Could you check a few things on this model? Use its own coordinates, in mm. Give positions to 0.01 mm unless a question says otherwise; leave off trailing zeros. Loops run counter-clockwise (first coordinate to the right, second up) from the corner with the lowest first, then second, coordinate; pieces in that order, holes last. Notation, with made-up numbers: M 50.25,9.5 L 72.25,9.5 A18 cw 72.25,21.5 Z; hole C 59.5,89.5 d4. An arc over 180 degrees is marked long. Return JSON: item names as keys, results as strings. Group by question number.
1. For pin 1 (3 mm diameter, centred on x = 4, y = 2.5, fed in from +Z); pin 2 (1.9 mm diameter, centred on y = 2.5, z = -3.5, fed in from -X); pin 3 (2 mm diameter, centred on y = 3, z = -106, fed in from +X); pin 4 (6.5 mm diameter, centred on x = 12.7, z = -203.2, fed in from +Y), each with a flat end and sliding along its axis, tell me the tip position at first contact or that it passes through.
2. If we section it at B-B (z = -111): Write out the boundary of the cut face in (x, y).
3. If we section it at C-C (x = 82): Write out the boundary of the cut face in (y, z).
4. If we section it at A-A (x = 12.7): Write out the boundary of the cut face in (y, z).
5. Please list where these lines run through material, in increasing order: line 1 (Z direction, x = 12.7, y = 2.5); line 2 (X direction, y = 5.5, z = -37); line 3 (Z direction, x = 57, y = 5.25).
```python
from build123d import *

# Parameters (mm, degrees)
SKETCH1_W           = 95.25
SKETCH1_H           = 215.9
BOSS_EXTRUDE1_DEPTH = 6.35
SKETCH2_W           = 6.35
SKETCH2_H           = 12.7
CUT_EXTRUDE1_DEPTH  = 7.35
LPATTERN1_COUNT     = 10
LPATTERN1_PITCH     = 25.4
SKETCH3_W           = 12.7
SKETCH3_H           = 6.35
CUT_EXTRUDE2_DEPTH  = 7.35
LPATTERN2_COUNT     = 2
LPATTERN2_PITCH     = 25.4
LPATTERN2_COL_COUNT = 3
LPATTERN2_COL_PITCH = 25.4
SKETCH4_R           = 3.571875
CUT_EXTRUDE3_DEPTH  = 7.35


with BuildPart() as part:
    # Sketch1 → Boss-Extrude1 (new body)
    with BuildSketch(Plane(origin=(0, 0, 0), x_dir=(1, 0, 0), z_dir=(0, 1, 0))):
        with Locations((47.625, 107.95)):
            Rectangle(SKETCH1_W, SKETCH1_H)
    extrude(amount=BOSS_EXTRUDE1_DEPTH)

    # Sketch2 → Cut-Extrude1 (cut, through all)
    with BuildSketch(Plane(origin=(0, 6.35, 0), x_dir=(1, 0, 0), z_dir=(0, 1, 0))):
        with Locations((3.175, 209.55)):
            Rectangle(SKETCH2_W, SKETCH2_H)
        with Locations((92.075, 209.55)):
            Rectangle(SKETCH2_W, SKETCH2_H)
    cut_extrude1 = extrude(amount=-CUT_EXTRUDE1_DEPTH, mode=Mode.SUBTRACT)

    # LPattern1: Cut-Extrude1 ×10
    with Locations(*[(0, 0, i * LPATTERN1_PITCH) for i in range(1, LPATTERN1_COUNT)]):
        add(cut_extrude1, mode=Mode.SUBTRACT)

    # Sketch3 → Cut-Extrude2 (cut, through all)
    with BuildSketch(Plane(origin=(0, 6.35, 0), x_dir=(1, 0, 0), z_dir=(0, 1, 0))):
        with Locations((34.925, 212.725)):
            Rectangle(SKETCH3_W, SKETCH3_H)
    cut_extrude2 = extrude(amount=-CUT_EXTRUDE2_DEPTH, mode=Mode.SUBTRACT)

    # LPattern2: Cut-Extrude2 ×2
    with Locations(*[(-i * LPATTERN2_PITCH, 0, 0) for i in range(1, LPATTERN2_COUNT)]):
        add(cut_extrude2, mode=Mode.SUBTRACT)

    # LPattern2 col: Cut-Extrude2 ×3
    with Locations(*[(i * LPATTERN2_COL_PITCH, 0, 0) for i in range(1, LPATTERN2_COL_COUNT)]):
        add(cut_extrude2, mode=Mode.SUBTRACT)

    # Sketch4 → Cut-Extrude3 (cut, through all)
    with BuildSketch(Plane(origin=(0, 6.35, 0), x_dir=(1, 0, 0), z_dir=(0, 1, 0))):
        with Locations((12.7, 203.2)):
            Circle(SKETCH4_R)
    extrude(amount=-CUT_EXTRUDE3_DEPTH, mode=Mode.SUBTRACT)


solid = part.part
```
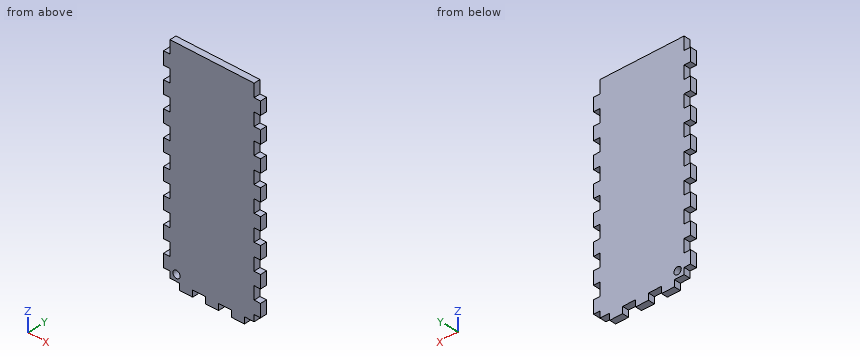
Answer:
{
 "1": {"pin 1": "stops at z = -12.7", "pin 2": "stops at x = 6.35", "pin 3": "stops at x = 88.9", "pin 4": "passes through"},
 "2": {"outline": "M 6.35,0 L 88.9,0 L 88.9,6.35 L 6.35,6.35 Z"},
 "3": {"outline": "M 0,-209.55 L 6.35,-209.55 L 6.35,0 L 0,0 Z"},
 "4": {"outline": "M 0,-209.55 L 6.35,-209.55 L 6.35,-206.77 L 0,-206.77 Z; M 0,-199.63 L 6.35,-199.63 L 6.35,0 L 0,0 Z"},
 "5": {"line 1": "z = -209.55 to -206.77, -199.63 to 0", "line 2": "x = 6.35 to 88.9", "line 3": "z = -209.55 to 0"}
}
